The model under review builds one solid part; all positions refer to its coordinate system, in mm. A direction names the side the tool comes from. Coordinates: 2 decimals unless noted, no trailing zeros. Loops run counter-clockwise (first coordinate to the right, second up) from the corner with the lowest first, then second, coordinate; pieces in that order, holes last. Notation, with made-up numbers: (-24.5, 48.25) - (21.5, 48.25) arc R24 cw to (21.5, 81.25) - close; hole circle Ø8 at (0.5, 59.25). An arc over 180 degrees is marked (long way). One line per item, written item: value. Start each with the question number.
1. For faces 1 (the face through (1.5, -3, 41.5)), 2 (the face through (5.8, 0.1, 20.7)), 3 (the face through (1, 0, 0)), 4 (the face through (1.26, 1.64, 35.18)), 5 (the face through (-5, -4.4, 10.1)), list the 3-axis set-ups (+Z, -Z, +X, -X, +Y, -Y) from which the entire face can be reached by the end or side of a thin tool; tool diameter is ignored.
2. Insertion check: P1, Ø3, axis at y = -4, z = 5.5, coming from the +X side; P2, Ø2.5, axis at x = 0, y = 0, coming from the -Z side; P3, Ø5, axis at y = -0.5, z = 4, coming from the -X side; P4, Ø2, axis at x = -5.5, z = 30.5, coming from the +Y side. Each pin has a flat end and moves straight along its axis. Give the tip position at first contact, or say it passes through.
3. Mouldability with a two-part tool opening along Y and no side actions: class faces 6 (the face through (3.763, -5.902, 25.071)), 7 (the face through (-6, 0, 21)), 8 (the face through (-0.137, -0.332, 28.974)), 9 (the face through (1.084, 3.715, 11.933)) as +Y half, -Y half, draft (parallel to the pull), parting line (faces both ways), or undercut.
4. We need section B-B, the plane z = 7. Give the boundary of the cut face in (x, y), then the cut area to 3 significant figures.
5. To check wall thickness, follow line 1 (Z direction, x = 4.25, y = 0); line 2 (Z direction, x = 5.75, y = -3.5); line 3 (Y direction, x = -1, z = 26.5). State the ranges of each line that lie inside material, in increasing order.
6. We need section A-A, the plane x = -5.5. Give the boundary of the cut face in (y, z).
7. We need section C-C, the plane y = -1.25. Count the separate pieces of the cut face and the enclosed holes in it, then the cut area to 3 significant figures.
Autodesk Inventor part; units mm, degrees
ref_plane "Arbeitsebene3" through (7, 0, 0) normal (1, 0, 0) x (0, 1, 0)
ref_plane "Arbeitsebene4" through (0, 7, 0) normal (0, 1, 0) x (-1, 0, 0)
ref_plane "XY Plane" through (0, 0, 0) normal (0, 0, 1) x (1, 0, 0)
sketch "Skizze1" plane through (0, 0, 0) normal (0, 0, 1) x (1, 0, 0)
  circle A0 centre (0, 0) radius 7
  dimension "d0" = 14
extrude "Extrusion1" add sketch "Skizze1" along normal blind 41.5
sketch "Skizze2" plane through (0, 0, 41.5) normal (0, 0, 1) x (1, 0, 0)
  circle A0 centre (0, 0) radius 7
hole "Bohrung1" at (0, 0, 41.5) direction (0, 0, -1) diameter 4.134 depth 11.5 tip angle 118
chamfer "Fasen1" distance 1 angle 45 1 edges at (0, 2.067, 41.5)
ref_plane "Arbeitsebene1" through (-7, 0, 0) normal (1, 0, 0) x (0, 1, 0)
ref_plane "Arbeitsebene2" through (0, -7, 0) normal (0, 1, 0) x (-1, 0, 0)
ref_plane "Arbeitsebene3" through (7, 0, 0) normal (1, 0, 0) x (0, 1, 0)
sketch "Skizze6" plane through (7, 0, 0) normal (1, 0, 0) x (0, 1, 0)
  line L0 (-7, 0) -> (-7, 41.5)
  line L1 (7, 0) -> (7, 41.5)
  line L2 (-7, 21.5) -> (7, 21.5)
  line L3 (7, 21.5) -> (7, 31.5)
  line L4 (7, 31.5) -> (-7, 31.5)
  line L5 (-7, 31.5) -> (-7, 21.5)
  line L6 (7, 41.5) -> (-7, 41.5)
  point P0 (0, 0)
  point P1 (-7, 31.5)
  point P2 (7, 21.5)
  dimension "d29" = 10
  dimension "d30" = 10
extrude "Extrusion4" cut sketch "Skizze6" against normal blind 2 contours L0 L4 L1 L2
sketch "Skizze7" plane through (5, 0, 0) normal (1, 0, 0) x (0, 0, -1)
  line L0 (-21.5, -4.899) -> (-21.5, 4.899)
  line L1 (0, 7) -> (0, -7)
  point P0 (0, 0)
  point P1 (-26.5, 0)
  point P2 (0, 0)
  point P3 (0, 0)
  point P4 (0, 0)
  dimension "d33" = 5
hole "Bohrung3" at (5, 0, 26.5) direction (-1, 0, 0) diameter 4.134 end through all
ref_plane "Arbeitsebene4" through (0, 7, 0) normal (0, 1, 0) x (-1, 0, 0)
sketch "Skizze8" plane through (0, 7, 0) normal (0, 1, 0) x (-1, 0, 0)
  line L0 (-5, 21.5) -> (-5, 21.5)
  line L1 (-5, 24.433) -> (-5, 28.567)
  line L2 (-5, 21.5) -> (-5, 31.5)
  line L3 (-5, 31.5) -> (-5, 21.5)
  line L4 (-5, 31.5) -> (-7, 31.5)
  line L5 (-5, 31.5) -> (-5, 21.5)
  line L6 (-5, 21.5) -> (-5, 31.5)
  line L7 (-5, 31.5) -> (-5, 31.5)
  line L8 (-7, 21.5) -> (-5, 21.5)
  line L9 (-5, 21.5) -> (-7, 19.5)
  line L10 (-7, 0) -> (-7, 41.5)
  line L11 (-5, 21.5) -> (-2.1716, 21.5) construction
  line L12 (-7, 19.5) -> (-7, 21.5)
  line L13 (-5, 31.5) -> (-7, 33.5)
  line L14 (-5, 31.5) -> (-2.1716, 31.5) construction
  line L15 (-7, 33.5) -> (-7, 31.5)
  point P0 (0, 0)
  dimension "d42" = 135
  dimension "d43" = 135
extrude "Extrusion5" cut sketch "Skizze8" against normal through all contours L9 L10 L8 | L4 L10 L13
sketch "Skizze9" plane through (-7, 0, 0) normal (1, 0, 0) x (0, 1, 0)
  line L0 (7, 0) -> (7, 41.5)
  line L1 (-7, 0) -> (-7, 41.5)
  line L2 (7, 0) -> (-7, 0)
  line L3 (-7, 0) -> (-7, 20)
  line L4 (-7, 20) -> (7, 20)
  line L5 (7, 20) -> (7, 0)
  point P0 (0, 0)
  point P1 (7, 20)
  dimension "d46" = 20
extrude "Extrusion6" cut sketch "Skizze9" along normal blind 2
sketch "Skizze10" plane through (0, -7, 0) normal (0, 1, 0) x (-1, 0, 0)
  line L0 (7, 20) -> (5, 20)
  line L1 (5, 20) -> (5, 20)
  line L2 (5, 20) -> (7, 22)
  line L3 (7, 20) -> (7, 41.5)
  line L4 (5, 20) -> (7.8284, 20) construction
  point P0 (0, 0)
  dimension "d49" = 45
extrude "Extrusion7" cut sketch "Skizze10" along normal through all
sketch "Skizze11" plane through (-5, 0, 0) normal (-1, 0, 0) x (0, 0, 1)
  line L0 (0, -4.899) -> (0, 4.899)
  point P0 (0, 0)
  point P1 (10, 0)
  point P2 (0, 0)
  point P3 (0, 0)
  dimension "d52" = 10
hole "Bohrung4" at (-5, 0, 10) direction (1, 0, 0) diameter 8.376 end through all
properties part number "TS_V1_Fallmagazin_Zylinderanbindung_int"
Findings below:
1. face 1: +Z, +X, -X, +Y, -Y
1. face 2: +X, +Y, -Y
1. face 3: -Z, +X, -X, +Y, -Y
1. face 4: +Z
1. face 5: -Z, -X, +Y, -Y
2. P1: x = 6.54
2. P2: z = 0
2. P3: x = -5
2. P4: y = 5.36
3. face 6: parting line
3. face 7: draft
3. face 8: undercut
3. face 9: undercut
4. outline: (-5, -4.9) arc R7 ccw to (6.36, -2.92) - (-5, -2.92) - close; (-5, 2.92) - (6.36, 2.92) arc R7 ccw to (-5, 4.9) - close
4. area: 71.5 mm2
5. line 1: 0 to 5.81, 14.19 to 24.43, 28.57 to 41.5
5. line 2: 0 to 7.7, 12.3 to 20.75, 32.25 to 41.5
5. line 3: -6.93 to -2.07, 2.07 to 6.93
6. outline: (-4.33, 20.5) - (4.33, 20.5) - (4.33, 41.5) - (-4.33, 41.5) - close; hole circle Ø4.13 at (0, 26.5)
7. separate pieces: 3
7. enclosed holes: 0
7. area: 335 mm2
